Geometry check sheet. Reference: the model listing, model coordinates, mm. Face numbers are marked on the shaded views. A direction names the side the tool comes from. Round coordinates to 2 decimals unless told otherwise and drop trailing zeros. Order: outer loops, then holes, each group sorted by start corner. A loop starts at its lowest first (then second) coordinate and runs counter-clockwise, first axis right, second up.
(1) Thickness scan on L1, parallel to Z at x = 91.74, y = 1.2 (3 decimals); L2, parallel to Y at x = 7, z = -12; L3, parallel to Z at x = 76, y = 6 (3 decimals). Record the ranges inside material, lowest first.
(2) Cross-section at D-D on x = 43. Enter the section's corners in (y, z) (3 decimals).
(3) Cross-section at C-C on z = -5.5. Enter the section's corners in (x, y), and give its area (3 significant figures).
(4) Gauge pin test, flat ends, axial feed: P1, Ø5, axis at x = 58, y = 6.5, coming from the -Z side (3 decimals); P2, Ø2, axis at x = 23.12, z = -3.008, coming from the -Y side; P3, Ø1.5, axis at x = 60, z = -13.5, coming from the -Y side; P4, Ø2.5, axis at x = 5.5, y = 16, coming from the -Z side. Record the tip position at first contact, or that the pin passes through.
(5) Cross-section at A-A on z = -24. Enter the section's corners in (x, y) (3 decimals).
(6) Set-up check for the marked faces 1, 2 and 3: record each of +Z, -Z, +X, -X, +Y, -Y from which the full face is reachable in a straight line by a thin tool's end or side.
(7) Draft check along X on the marked faces 4 and 5. Enter one of: pulls with the +X half, pulls with the -X half, needs draft (parallel to the pull), parting line crosses it, or undercut.
(8) Cross-section at B-B on x = 79.12. Enter the section's corners in (y, z) (3 decimals), and give its area (3 significant figures).
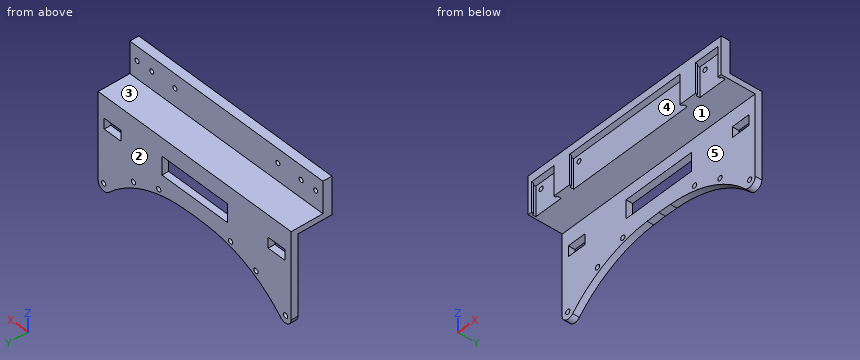
from build123d import *

# Parameters (mm, degrees)
BOSS_EXTRUDE2_DEPTH = 14.285
SKETCH4_W           = 105.034
SKETCH4_H           = 3.81
BOSS_EXTRUDE3_DEPTH = 19.533
SKETCH5_W           = 15.24
SKETCH5_H           = 15.24
CUT_EXTRUDE1_DEPTH  = 105.034
BOSS_EXTRUDE7_START = -3.175
BOSS_EXTRUDE7_DEPTH = 3.175
CUT_EXTRUDE2_REACH  = 21.533
SKETCH9_R           = 1.15
SKETCH9_W           = 35.56
SKETCH9_H           = 8.89
SKETCH9_W_2         = 9.19
SKETCH9_H_2         = 5.08
CUT_EXTRUDE3_REACH  = 6.293
SKETCH13_R          = 1.0922


with BuildPart() as part:
    # Sketch1 → Boss-Extrude2 (new body)
    with BuildSketch(Plane.XY):
        Polygon((13.381, 0.381), (-0.381, 0.381), (-0.381, -1.397), (0.4572, -1.397), (0.4572, -2.413), (-1.397, -2.413), (-1.397, 1.397), (-1.397, 17.12), (103.637, 17.12), (103.637, 1.397), (103.637, -2.413), (101.7828, -2.413), (101.7828, -1.397), (102.621, -1.397), (102.621, 0.381), (88.859, 0.381), (88.859, -1.397), (89.621, -1.397), (89.621, -2.413), (87.843, -2.413), (83.017, -2.413), (81.1628, -2.413), (81.1628, -1.397), (82.001, -1.397), (82.001, 0.381), (20.239, 0.381), (20.239, -1.397), (21.0772, -1.397), (21.0772, -2.413), (19.223, -2.413), (14.397, -2.413), (12.619, -2.413), (12.619, -1.397), (13.381, -1.397), align=None)
    extrude(amount=-BOSS_EXTRUDE2_DEPTH)

    # Sketch4 → Boss-Extrude3 (add)
    with BuildSketch(Plane(origin=(0, 17.12, 0), x_dir=(1, 0, 0), z_dir=(0, 1, 0))):
        with Locations((51.12, -1.905)):
            Rectangle(SKETCH4_W, SKETCH4_H)
    extrude(amount=-BOSS_EXTRUDE3_DEPTH)

    # Sketch5 → Cut-Extrude1 (cut)
    with BuildSketch(Plane(origin=(103.637, 0, 0), x_dir=(0, 0, -1), z_dir=(1, 0, 0))):
        with Locations((3.81, 9.5)):
            Rectangle(SKETCH5_W, SKETCH5_H)
    extrude(amount=-CUT_EXTRUDE1_DEPTH, mode=Mode.SUBTRACT)

    # Sketch8 → Boss-Extrude7 (add)
    with BuildSketch(Plane(origin=(0, 17.12, 0), x_dir=(1, 0, 0), z_dir=(0, 1, 0)).offset(BOSS_EXTRUDE7_START)):
        with BuildLine():
            Line((-1.397, 52.90899931), (-1.397, 14.285))
            Line((-1.397, 14.285), (103.637, 14.285))
            Line((103.637, 14.285), (103.637, 52.90899931))
            ThreePointArc((103.637, 52.90899931), (101.565258526, 55.97325582), (97.949738971, 55.192359514))
            ThreePointArc((97.949738971, 55.192359514), (79.465238701, 42.200806947), (57.433563247, 37.194564339))
            Line((57.433563247, 37.194564339), (51.12, 37.012430992))
            Line((51.12, 37.012430992), (44.806436753, 37.194564339))
            ThreePointArc((44.806436753, 37.194564339), (22.774761299, 42.200806947), (4.290261029, 55.192359514))
            ThreePointArc((4.290261029, 55.192359514), (0.674741474, 55.97325582), (-1.397, 52.90899931))
        make_face()
    extrude(amount=BOSS_EXTRUDE7_DEPTH)

    # Sketch9 → Cut-Extrude2 (cut, up to next)
    with BuildSketch(Plane(origin=(0, 17.12, 0), x_dir=(1, 0, 0), z_dir=(0, 1, 0)), mode=Mode.PRIVATE) as cut_extrude2_sk1:
        with Locations((100.617474683, 52.660280557)):
            Circle(SKETCH9_R)
    cut_extrude2_tool1 = extrude(cut_extrude2_sk1.sketch, amount=-CUT_EXTRUDE2_REACH, mode=Mode.PRIVATE) & part.part
    add(cut_extrude2_tool1.solids().sort_by_distance((100.617475, 17.12, -52.660281))[0], mode=Mode.SUBTRACT)
    # Sketch9 → Cut-Extrude2 (cut, up to next)
    with BuildSketch(Plane(origin=(0, 17.12, 0), x_dir=(1, 0, 0), z_dir=(0, 1, 0)), mode=Mode.PRIVATE) as cut_extrude2_sk2:
        with Locations((84.44065509, 41.851275276)):
            Circle(SKETCH9_R)
    cut_extrude2_tool2 = extrude(cut_extrude2_sk2.sketch, amount=-CUT_EXTRUDE2_REACH, mode=Mode.PRIVATE) & part.part
    add(cut_extrude2_tool2.solids().sort_by_distance((84.440655, 17.12, -41.851275))[0], mode=Mode.SUBTRACT)
    # Sketch9 → Cut-Extrude2 (cut, up to next)
    with BuildSketch(Plane(origin=(0, 17.12, 0), x_dir=(1, 0, 0), z_dir=(0, 1, 0)), mode=Mode.PRIVATE) as cut_extrude2_sk3:
        with Locations((70.655700553, 36.645378632)):
            Circle(SKETCH9_R)
    cut_extrude2_tool3 = extrude(cut_extrude2_sk3.sketch, amount=-CUT_EXTRUDE2_REACH, mode=Mode.PRIVATE) & part.part
    add(cut_extrude2_tool3.solids().sort_by_distance((70.655701, 17.12, -36.645379))[0], mode=Mode.SUBTRACT)
    # Sketch9 → Cut-Extrude2 (cut, up to next)
    with BuildSketch(Plane(origin=(0, 17.12, 0), x_dir=(1, 0, 0), z_dir=(0, 1, 0)), mode=Mode.PRIVATE) as cut_extrude2_sk4:
        with Locations((31.584299447, 36.645378632)):
            Circle(SKETCH9_R)
    cut_extrude2_tool4 = extrude(cut_extrude2_sk4.sketch, amount=-CUT_EXTRUDE2_REACH, mode=Mode.PRIVATE) & part.part
    add(cut_extrude2_tool4.solids().sort_by_distance((31.584299, 17.12, -36.645379))[0], mode=Mode.SUBTRACT)
    # Sketch9 → Cut-Extrude2 (cut, up to next)
    with BuildSketch(Plane(origin=(0, 17.12, 0), x_dir=(1, 0, 0), z_dir=(0, 1, 0)), mode=Mode.PRIVATE) as cut_extrude2_sk5:
        with Locations((17.79934491, 41.851275276)):
            Circle(SKETCH9_R)
    cut_extrude2_tool5 = extrude(cut_extrude2_sk5.sketch, amount=-CUT_EXTRUDE2_REACH, mode=Mode.PRIVATE) & part.part
    add(cut_extrude2_tool5.solids().sort_by_distance((17.799345, 17.12, -41.851275))[0], mode=Mode.SUBTRACT)
    # Sketch9 → Cut-Extrude2 (cut, up to next)
    with BuildSketch(Plane(origin=(0, 17.12, 0), x_dir=(1, 0, 0), z_dir=(0, 1, 0)), mode=Mode.PRIVATE) as cut_extrude2_sk6:
        with Locations((1.622525317, 52.660280557)):
            Circle(SKETCH9_R)
    cut_extrude2_tool6 = extrude(cut_extrude2_sk6.sketch, amount=-CUT_EXTRUDE2_REACH, mode=Mode.PRIVATE) & part.part
    add(cut_extrude2_tool6.solids().sort_by_distance((1.622525, 17.12, -52.660281))[0], mode=Mode.SUBTRACT)
    # Sketch9 → Cut-Extrude2 (cut, up to next)
    with BuildSketch(Plane(origin=(0, 17.12, 0), x_dir=(1, 0, 0), z_dir=(0, 1, 0)), mode=Mode.PRIVATE) as cut_extrude2_sk7:
        with Locations((51.1199898, 24.445)):
            Rectangle(SKETCH9_W, SKETCH9_H)
    cut_extrude2_tool7 = extrude(cut_extrude2_sk7.sketch, amount=-CUT_EXTRUDE2_REACH, mode=Mode.PRIVATE) & part.part
    add(cut_extrude2_tool7.solids().sort_by_distance((51.11999, 17.12, -24.445))[0], mode=Mode.SUBTRACT)
    # Sketch9 → Cut-Extrude2 (cut, up to next)
    with BuildSketch(Plane(origin=(0, 17.12, 0), x_dir=(1, 0, 0), z_dir=(0, 1, 0)), mode=Mode.PRIVATE) as cut_extrude2_sk8:
        with Locations((6.5, 24.445)):
            Rectangle(SKETCH9_W_2, SKETCH9_H_2)
    cut_extrude2_tool8 = extrude(cut_extrude2_sk8.sketch, amount=-CUT_EXTRUDE2_REACH, mode=Mode.PRIVATE) & part.part
    add(cut_extrude2_tool8.solids().sort_by_distance((6.5, 17.12, -24.445))[0], mode=Mode.SUBTRACT)
    # Sketch9 → Cut-Extrude2 (cut, up to next)
    with BuildSketch(Plane(origin=(0, 17.12, 0), x_dir=(1, 0, 0), z_dir=(0, 1, 0)), mode=Mode.PRIVATE) as cut_extrude2_sk9:
        with Locations((95.74, 24.445)):
            Rectangle(SKETCH9_W_2, SKETCH9_H_2)
    cut_extrude2_tool9 = extrude(cut_extrude2_sk9.sketch, amount=-CUT_EXTRUDE2_REACH, mode=Mode.PRIVATE) & part.part
    add(cut_extrude2_tool9.solids().sort_by_distance((95.74, 17.12, -24.445))[0], mode=Mode.SUBTRACT)

    # Sketch13 → Cut-Extrude3 (cut, up to next)
    with BuildSketch(Plane(origin=(0, 1.88, 0), x_dir=(1, 0, 0), z_dir=(0, 1, 0)), mode=Mode.PRIVATE) as cut_extrude3_sk1:
        with Locations((23.12, 3.008)):
            Circle(SKETCH13_R)
    cut_extrude3_tool1 = extrude(cut_extrude3_sk1.sketch, amount=-CUT_EXTRUDE3_REACH, mode=Mode.PRIVATE) & part.part
    add(cut_extrude3_tool1.solids().sort_by_distance((23.12, 1.88, -3.008))[0], mode=Mode.SUBTRACT)
    # Sketch13 → Cut-Extrude3 (cut, up to next)
    with BuildSketch(Plane(origin=(0, 1.88, 0), x_dir=(1, 0, 0), z_dir=(0, 1, 0)), mode=Mode.PRIVATE) as cut_extrude3_sk2:
        with Locations((10.5, 3.008)):
            Circle(SKETCH13_R)
    cut_extrude3_tool2 = extrude(cut_extrude3_sk2.sketch, amount=-CUT_EXTRUDE3_REACH, mode=Mode.PRIVATE) & part.part
    add(cut_extrude3_tool2.solids().sort_by_distance((10.5, 1.88, -3.008))[0], mode=Mode.SUBTRACT)
    # Sketch13 → Cut-Extrude3 (cut, up to next)
    with BuildSketch(Plane(origin=(0, 1.88, 0), x_dir=(1, 0, 0), z_dir=(0, 1, 0)), mode=Mode.PRIVATE) as cut_extrude3_sk3:
        with Locations((2.5, 3.008)):
            Circle(SKETCH13_R)
    cut_extrude3_tool3 = extrude(cut_extrude3_sk3.sketch, amount=-CUT_EXTRUDE3_REACH, mode=Mode.PRIVATE) & part.part
    add(cut_extrude3_tool3.solids().sort_by_distance((2.5, 1.88, -3.008))[0], mode=Mode.SUBTRACT)
    # Sketch13 → Cut-Extrude3 (cut, up to next)
    with BuildSketch(Plane(origin=(0, 1.88, 0), x_dir=(1, 0, 0), z_dir=(0, 1, 0)), mode=Mode.PRIVATE) as cut_extrude3_sk4:
        with Locations((79.12, 3.008)):
            Circle(SKETCH13_R)
    cut_extrude3_tool4 = extrude(cut_extrude3_sk4.sketch, amount=-CUT_EXTRUDE3_REACH, mode=Mode.PRIVATE) & part.part
    add(cut_extrude3_tool4.solids().sort_by_distance((79.12, 1.88, -3.008))[0], mode=Mode.SUBTRACT)
    # Sketch13 → Cut-Extrude3 (cut, up to next)
    with BuildSketch(Plane(origin=(0, 1.88, 0), x_dir=(1, 0, 0), z_dir=(0, 1, 0)), mode=Mode.PRIVATE) as cut_extrude3_sk5:
        with Locations((91.74, 3.008)):
            Circle(SKETCH13_R)
    cut_extrude3_tool5 = extrude(cut_extrude3_sk5.sketch, amount=-CUT_EXTRUDE3_REACH, mode=Mode.PRIVATE) & part.part
    add(cut_extrude3_tool5.solids().sort_by_distance((91.74, 1.88, -3.008))[0], mode=Mode.SUBTRACT)
    # Sketch13 → Cut-Extrude3 (cut, up to next)
    with BuildSketch(Plane(origin=(0, 1.88, 0), x_dir=(1, 0, 0), z_dir=(0, 1, 0)), mode=Mode.PRIVATE) as cut_extrude3_sk6:
        with Locations((99.74, 3.008)):
            Circle(SKETCH13_R)
    cut_extrude3_tool6 = extrude(cut_extrude3_sk6.sketch, amount=-CUT_EXTRUDE3_REACH, mode=Mode.PRIVATE) & part.part
    add(cut_extrude3_tool6.solids().sort_by_distance((99.74, 1.88, -3.008))[0], mode=Mode.SUBTRACT)


solid = part.part
Found:
1. L1: z = -14.285 to -4.1, -1.916 to 3.81
1. L2: y = 0.38 to 17.12
1. L3: z = -14.285 to -11.43
2. outline: (-2.413, 0) - (0.381, 0) - (0.381, -14.285) - (13.945, -14.285) - (13.945, -20) - (17.12, -20) - (17.12, -11.43) - (1.88, -11.43) - (1.88, 3.81) - (-2.413, 3.81) - close; (13.945, -37.275) - (17.12, -37.275) - (17.12, -28.89) - (13.945, -28.89) - close
3. outline: (-1.4, -2.41) - (0.46, -2.41) - (0.46, -1.4) - (-0.38, -1.4) - (-0.38, 0.38) - (13.38, 0.38) - (13.38, -1.4) - (12.62, -1.4) - (12.62, -2.41) - (21.08, -2.41) - (21.08, -1.4) - (20.24, -1.4) - (20.24, 0.38) - (82, 0.38) - (82, -1.4) - (81.16, -1.4) - (81.16, -2.41) - (89.62, -2.41) - (89.62, -1.4) - (88.86, -1.4) - (88.86, 0.38) - (102.62, 0.38) - (102.62, -1.4) - (101.78, -1.4) - (101.78, -2.41) - (103.64, -2.41) - (103.64, 1.88) - (-1.4, 1.88) - close
3. area: 206 mm2
4. P1: stops at z = -14.285
4. P2: passes through
4. P3: stops at y = 0.38
4. P4: stops at z = -55.23
5. outline: (-1.397, 13.945) - (1.905, 13.945) - (1.905, 17.12) - (-1.397, 17.12) - close; (11.095, 13.945) - (33.34, 13.945) - (33.34, 17.12) - (11.095, 17.12) - close; (68.9, 13.945) - (91.145, 13.945) - (91.145, 17.12) - (68.9, 17.12) - close; (100.335, 13.945) - (103.637, 13.945) - (103.637, 17.12) - (100.335, 17.12) - close
6. face 1: -Z, +X, -X, -Y
6. face 2: +Z, -Z, +X, -X, +Y
6. face 3: +Z, +X, -X, +Y
7. face 4: undercut
7. face 5: needs draft
8. outline: (-2.413, 0) - (0.381, 0) - (0.381, -1.916) - (1.88, -1.916) - (1.88, 3.81) - (-2.413, 3.81) - close; (0.381, -14.285) - (13.945, -14.285) - (13.945, -42.049) - (17.12, -42.049) - (17.12, -11.43) - (1.88, -11.43) - (1.88, -4.1) - (0.381, -4.1) - close
8. area: 166 mm2
